Design review of the part built by this model. Coordinates are the model's own, in mm. Face numbers are marked on the shaded views. A direction names the side the tool comes from. Coordinates: 2 decimals unless noted, no trailing zeros. Loops run counter-clockwise (first coordinate to the right, second up) from the corner with the lowest first, then second, coordinate; pieces in that order, holes last. Notation, with made-up numbers: (-0.75, -37) - (57.25, -37) arc R25 cw to (57.25, -22) - close; hole circle Ø10 at (3, -13). An arc over 180 degrees is marked (long way). Return JSON: item names as keys, results as strings. Group by question number.
from build123d import *

# Parameters (mm, degrees)
F0_R     = 3.6
F1_DEPTH = 3
F2_DEPTH = 10
F3_DEPTH = 15


with BuildPart() as f1:
    # F0 (on Front) → F1 (new body)
    with BuildSketch(Plane.XZ):
        with BuildLine():
            ThreePointArc((15.5, 12.5), (14.62132, 14.62132), (12.5, 15.5))
            Line((12.5, 15.5), (-12.5, 15.5))
            ThreePointArc((-12.5, 15.5), (-14.62132, 14.62132), (-15.5, 12.5))
            Line((-15.5, 12.5), (-15.5, -12.5))
            ThreePointArc((-15.5, -12.5), (-14.62132, -14.62132), (-12.5, -15.5))
            Line((-12.5, -15.5), (12.5, -15.5))
            ThreePointArc((12.5, -15.5), (14.62132, -14.62132), (15.5, -12.5))
            Line((15.5, -12.5), (15.5, 12.5))
        make_face()
        Circle(F0_R, mode=Mode.SUBTRACT)
    extrude(amount=F1_DEPTH)

    # F0 (on Front) → F2 (join)
    with BuildSketch(Plane.XZ):
        Circle(F0_R)
    extrude(amount=F2_DEPTH)

    # F0 (on Front) → F3 (join)
    with BuildSketch(Plane.XZ):
        with BuildLine():
            Line((14, 17), (-14, 17))
            ThreePointArc((-14, 17), (-16.12132, 16.12132), (-17, 14))
            Line((-17, 14), (-17, -14))
            ThreePointArc((-17, -14), (-16.12132, -16.12132), (-14, -17))
            Line((-14, -17), (14, -17))
            ThreePointArc((14, -17), (16.12132, -16.12132), (17, -14))
            Line((17, -14), (17, 14))
            ThreePointArc((17, 14), (16.12132, 16.12132), (14, 17))
        make_face()
        with BuildLine():
            Line((-12.5, 15.5), (12.5, 15.5))
            ThreePointArc((12.5, 15.5), (14.62132, 14.62132), (15.5, 12.5))
            Line((15.5, 12.5), (15.5, -12.5))
            ThreePointArc((15.5, -12.5), (14.62132, -14.62132), (12.5, -15.5))
            Line((12.5, -15.5), (-12.5, -15.5))
            ThreePointArc((-12.5, -15.5), (-14.62132, -14.62132), (-15.5, -12.5))
            Line((-15.5, -12.5), (-15.5, 12.5))
            ThreePointArc((-15.5, 12.5), (-14.62132, 14.62132), (-12.5, 15.5))
        make_face(mode=Mode.SUBTRACT)
    extrude(amount=F3_DEPTH)


solid = f1.part
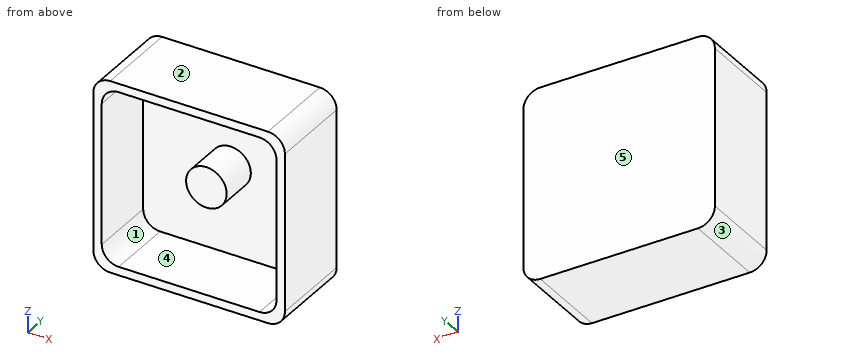
Item 1: Add section D-D (z = 9). State the section outline as (x, y) points, then the cut area to 3 significant figures.
Item 2: For P1, Ø4, axis at x = -9, z = -9, coming from the -Y side; P2, Ø3.5, axis at x = 0, z = -1, coming from the -Y side, all flat-tipped, find the tip position at first contact; note any pin that passes through.
Item 3: Add section B-B (x = 5). State the section outline as (y, z) points, then the cut area to 3 significant figures.
Item 4: Draft analysis for pull direction Z (two halves, no side actions). For the marked faces 3, 4 and 5, state which applies: pulls with the +Z half, pulls with the -Z half, needs draft (parallel to the pull), parting line crosses it, or undercut.
Item 5: For the marked faces 1 and 2, list the 3-axis set-ups (+Z, -Z, +X, -X, +Y, -Y) from which the entire face can be reached by the end or side of a thin tool; tool diameter is ignored.
Item 6: To check wall thickness, follow line 1 (X direction, y = -12.5, z = 5); line 2 (X direction, y = -6.5, z = 2). State the ranges of each line that lie inside material, in increasing order. Write a range as from..to.
Item 7: Add section A-A (y = -5.5). State the section outline as (x, z) points.
Item 8: Add section C-C (y = -13.25). State the section outline as (x, z) points.
Answers below:
{
 "1": {"outline": "(-17, -15) - (-15.5, -15) - (-15.5, -3) - (15.5, -3) - (15.5, -15) - (17, -15) - (17, 0) - (-17, 0) - close", "area": "138 mm^2"},
 "2": {"P1": "stops at y = -3", "P2": "stops at y = -10"},
 "3": {"outline": "(-15, -17) - (0, -17) - (0, 17) - (-15, 17) - (-15, 15.5) - (-3, 15.5) - (-3, -15.5) - (-15, -15.5) - close", "area": "138 mm^2"},
 "4": {"face 3": "pulls with the -Z half", "face 4": "undercut", "face 5": "needs draft"},
 "5": {"face 1": "-Y", "face 2": "+Z, +X, -X, +Y, -Y"},
 "6": {"line 1": "x = -17..-15.5, 15.5..17", "line 2": "x = -17..-15.5, -2.99..2.99, 15.5..17"},
 "7": {"outline": "(-17, -14) arc R3 ccw to (-14, -17) - (14, -17) arc R3 ccw to (17, -14) - (17, 14) arc R3 ccw to (14, 17) - (-14, 17) arc R3 ccw to (-17, 14) - close; circle Ø7.2 at (0, 0); hole (-15.5, -12.5) arc R3 ccw to (-12.5, -15.5) - (12.5, -15.5) arc R3 ccw to (15.5, -12.5) - (15.5, 12.5) arc R3 ccw to (12.5, 15.5) - (-12.5, 15.5) arc R3 ccw to (-15.5, 12.5) - close"},
 "8": {"outline": "(-17, -14) arc R3 ccw to (-14, -17) - (14, -17) arc R3 ccw to (17, -14) - (17, 14) arc R3 ccw to (14, 17) - (-14, 17) arc R3 ccw to (-17, 14) - close; hole (-15.5, -12.5) arc R3 ccw to (-12.5, -15.5) - (12.5, -15.5) arc R3 ccw to (15.5, -12.5) - (15.5, 12.5) arc R3 ccw to (12.5, 15.5) - (-12.5, 15.5) arc R3 ccw to (-15.5, 12.5) - close"}
}
